The figure shows three views and two pictorial views of one solid part (mm, origin at its lowest corner). Answer the questions. Round coordinates to 2 decimals unless told otherwise and drop trailing zeros. Loops run counter-clockwise (first coordinate to the right, second up) from the corner with the lowest first, then second, coordinate; pieces in that order, holes last. Notation, with made-up numbers: (20, 88.5) -> (69, 88.5) arc R6 ccw to (69, 99.5) -> close; hole circle Ø4 at (-12, 11.25). An arc over 180 degrees is marked (long way). Use a Markdown table: item, result. Add a question column.
Q1. Consider line 1 (Y direction, x = 17.2, z = 0.4); line 2 (X direction, y = 4, z = 0.8). Determine where each line is inside the solid, lowest interval first.
Q2. Section A-A on y = 2.8 is taken. Give the vertices of the cut face in (x, z), then the cut area to 3 significant figures.
Q3. Section B-B on z = 0.35 is taken. Give the vertices of the cut face in (x, y), then the cut area to 3 significant figures.
Q4. Section C-C on x = 2.8 is taken. Give the vertices of the cut face in (y, z), then the cut area to 3 significant figures.
Q5. For a pull along Z with two mould halves and no side action, classify the marked faces 1 and 2 as released by +Z, released by -Z, zero draft, split by the parting line, or undercut.
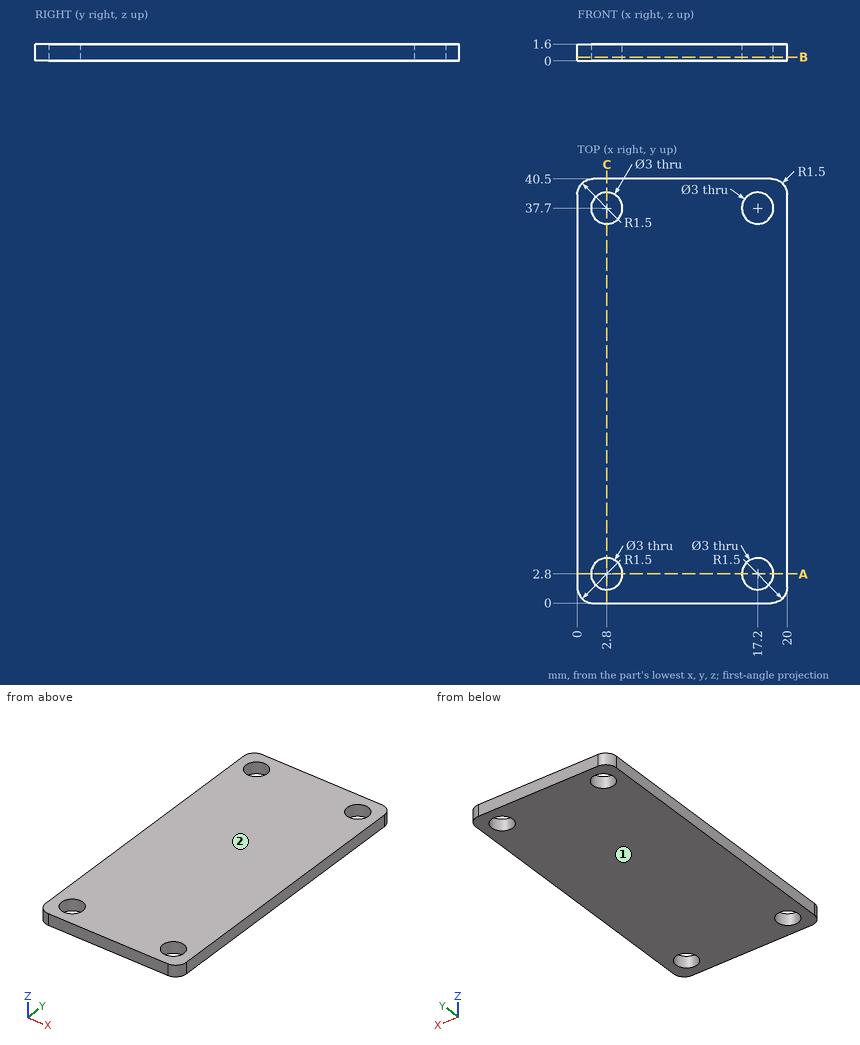
Checked values:
| question | item | result |
|---|---|---|
| 1 | line 1 | y = 0 to 1.3, 4.3 to 36.2, 39.2 to 40.5 |
| 1 | line 2 | x = 0 to 1.9, 3.7 to 16.3, 18.1 to 20 |
| 2 | outline | (0, 0) -> (1.3, 0) -> (1.3, 1.6) -> (0, 1.6) -> close; (4.3, 0) -> (15.7, 0) -> (15.7, 1.6) -> (4.3, 1.6) -> close; (18.7, 0) -> (20, 0) -> (20, 1.6) -> (18.7, 1.6) -> close |
| 2 | area | 22.4 mm2 |
| 3 | outline | (0, 1.5) arc R1.5 ccw to (1.5, 0) -> (18.5, 0) arc R1.5 ccw to (20, 1.5) -> (20, 39) arc R1.5 ccw to (18.5, 40.5) -> (1.5, 40.5) arc R1.5 ccw to (0, 39) -> close; hole circle Ø3 at (2.8, 2.8); hole circle Ø3 at (2.8, 37.7); hole circle Ø3 at (17.2, 2.8); hole circle Ø3 at (17.2, 37.7) |
| 3 | area | 780 mm2 |
| 4 | outline | (0, 0) -> (1.3, 0) -> (1.3, 1.6) -> (0, 1.6) -> close; (4.3, 0) -> (36.2, 0) -> (36.2, 1.6) -> (4.3, 1.6) -> close; (39.2, 0) -> (40.5, 0) -> (40.5, 1.6) -> (39.2, 1.6) -> close |
| 4 | area | 55.2 mm2 |
| 5 | face 1 | released by -Z |
| 5 | face 2 | released by +Z |
